Could you check a few things on this model? Use its own coordinates, in mm. A direction names the side the tool comes from. Give positions to 0.01 mm unless a question says otherwise; leave off trailing zeros. Write each loop counter-clockwise with the first axis right and the second up, starting at its lowest first coordinate (ties: lowest second). Pieces come first, ordered by that corner, then holes. Notation, with made-up numbers: (48.25, 60.5) - (59.25, 60.5) arc R25 ccw to (59.25, 90.5) - close; hole circle Ø9 at (41.25, -8). An arc over 180 degrees is marked (long way). Answer as CSV lines item,"result". Start each with the question number.
Q1. If I drill on line 1 along Z through (x, y) = (0, 1.4); line 2 along Y through (x, z) = (-8.7, 0); line 3 along Z through (x, y) = (0, 12), over which ranges is the centre line in solid material (lowest first)?
Q2. Imagine slicing it at D-D on x = -4. List the corners of the cut face in (y, z) for me.
Q3. Imagine slicing it at C-C on z = 13. List the corners of the cut face in (x, y) for me.
Q4. We'd pull the mould along X, two halves only. Please class faces 3 (the face through (-7.348, 8.536, 0.325)), 4 (the face through (9.237, 9.93, 3.83)), 5 (the face through (-0.325, 8.536, -7.346)): pulls with the +X half, pulls with the -X half, needs draft (parallel to the pull), parting line crosses it, or undercut.
Q5. Imagine slicing it at B-B on y = 11. List the corners of the cut face in (x, z) for me, and give its area (3 significant figures).
Q6. Will these pins go through, and if not, where does the flat tip stop? pin 1 Ø1 at (y, z) = (4.5, 10.5) entering from -X; pin 2 Ø2 at (y, z) = (12.5, -7.5) entering from +X; pin 3 Ø5 at (x, y) = (9, 5) entering from +Z; pin 4 Ø2.5 at (x, z) = (0, 13.75) entering from +Y.
Q7. Imagine slicing it at A-A on x = 0. List the corners of the cut face in (y, z) for me, and give its area (3 significant figures).
Q8. On a 3-axis mill with a long thin cutter (end or side, diameter ignored), from which of +Z, -Z, +X, -X, +Y, -Y can I reach the whole of each face in a straight line? I mean faces 1 (the face through (8, 5, 8)), 2 (the face through (4, 0, 4)). Say none if no direction works.
```python
from build123d import *

# Parameters (mm, degrees)
ESBO_O1_R                = 17.5
RESSALTO_EXTRUS_O1_DEPTH = 5
ESBO_O2_R                = 10
RESSALTO_EXTRUS_O2_DEPTH = 10
ESBO_O3_R                = 5
CORTE_EXTRUS_O1_DEPTH    = 16
ESBO_O4_R                = 1.5
CORTE_EXTRUS_O2_DEPTH    = 10
ESBO_O5_R                = 1.5
CORTE_EXTRUS_O3_DEPTH    = 18.5
ESBO_O6_R                = 1.5
CORTE_EXTRUS_O4_DEPTH    = 10


with BuildPart() as part:
    # Esboço1 → Ressalto-extrusão1 (new body)
    with BuildSketch(Plane(origin=(0, 0, 0), x_dir=(1, 0, 0), z_dir=(0, 1, 0))):
        Circle(ESBO_O1_R)
    extrude(amount=RESSALTO_EXTRUS_O1_DEPTH)

    # Esboço2 → Ressalto-extrusão2 (add)
    with BuildSketch(Plane(origin=(0, 5, 0), x_dir=(1, 0, 0), z_dir=(0, 1, 0))):
        Circle(ESBO_O2_R)
    extrude(amount=RESSALTO_EXTRUS_O2_DEPTH)

    # Esboço3 → Corte-extrusão1 (cut, through all)
    with BuildSketch(Plane(origin=(0, 15, 0), x_dir=(1, 0, 0), z_dir=(0, 1, 0))):
        Circle(ESBO_O3_R)
    extrude(amount=-CORTE_EXTRUS_O1_DEPTH, mode=Mode.SUBTRACT)

    # Esboço4 → Corte-extrusão2 (cut)
    with BuildSketch(Plane(origin=(0, 5, 0), x_dir=(1, 0, 0), z_dir=(0, 1, 0))):
        with Locations((0, 13.75)):
            Circle(ESBO_O4_R)
        with Locations((0, -13.75)):
            Circle(ESBO_O4_R)
    extrude(amount=-CORTE_EXTRUS_O2_DEPTH, mode=Mode.SUBTRACT)

    # Esboço5 → Corte-extrusão3 (cut, through all)
    with BuildSketch(Plane.XY):
        with Locations((0, 10)):
            Circle(ESBO_O5_R)
    extrude(amount=-CORTE_EXTRUS_O3_DEPTH, mode=Mode.SUBTRACT)

    # Esboço6 → Corte-extrusão4 (cut)
    with BuildSketch(Plane(origin=(0, 0, 0), x_dir=(0, 0, -1), z_dir=(1, 0, 0))):
        with Locations((0, 10)):
            Circle(ESBO_O6_R)
    extrude(amount=-CORTE_EXTRUS_O4_DEPTH, mode=Mode.SUBTRACT)


solid = part.part
```
Conclusion:
1,line 1,"-17.5 to -15.25, -12.25 to -5, 5 to 12.25, 15.25 to 17.5"
1,line 2,"0 to 8.5, 11.5 to 15"
1,line 3,"-10 to -5, 5 to 10"
2,outline,"(0, -17.04) - (5, -17.04) - (5, -9.17) - (15, -9.17) - (15, -3) - (0, -3) - close; (0, 3) - (15, 3) - (15, 9.17) - (5, 9.17) - (5, 17.04) - (0, 17.04) - close"
3,outline,"(-11.72, 0) - (-1.3, 0) - (-1.3, 5) - (-11.72, 5) - close; (1.3, 0) - (11.72, 0) - (11.72, 5) - (1.3, 5) - close"
4,face 3,"needs draft"
4,face 4,"parting line crosses it"
4,face 5,"undercut"
5,outline,"(-9.94, -1.12) arc R10 ccw to (-1.12, -9.94) - (-1.12, -4.87) arc R5 cw to (-4.87, -1.12) - close; (-9.94, 1.12) - (-4.87, 1.12) arc R5 cw (long way) to (1.12, -4.87) - (1.12, -9.94) arc R10 ccw (long way) to start"
5,area,"213 mm^2"
6,pin 1,"x = -14.36"
6,pin 2,"x = 7.6"
6,pin 3,"z = 16.25"
6,pin 4,"through"
7,outline,"(0, -17.5) - (5, -17.5) - (5, -15.25) - (0, -15.25) - close; (0, -12.25) - (5, -12.25) - (5, -10) - (8.5, -10) - (8.5, -5) - (0, -5) - close; (0, 5) - (15, 5) - (15, 10) - (5, 10) - (5, 12.25) - (0, 12.25) - close; (0, 15.25) - (5, 15.25) - (5, 17.5) - (0, 17.5) - close; (11.5, -10) - (15, -10) - (15, -5) - (11.5, -5) - close"
7,area,"180 mm^2"
8,face 1,"+Y"
8,face 2,"+Z, -Z, +X, -X, -Y"
